Could you check a few things on this model? Use its own coordinates, in mm. A direction names the side the tool comes from. Give positions to 0.01 mm unless a question says otherwise; leave off trailing zeros. Order: outer loops, then holes, each group sorted by start corner. A loop starts at its lowest first (then second) coordinate and runs counter-clockwise, first axis right, second up. Notation, with made-up numbers: (86.5, -15.75) - (122.5, -15.75) arc R17 ccw to (122.5, -5.75) - close; hole circle Ø4 at (44, 57.25). An arc over 180 degrees is marked (long way). One line per question, with ' | ' between items. Start each with the question number.
1. Which directions (+Z, -Z, +X, -X, +Y, -Y) give clear straight access to the entire face, cutting with the end or side of a thin tool? Please do faces 4 (the cylindrical face through (-1.08, -4.88, 0.25)), 5 (the flat face through (6, 0, 3.5)), 6 (the cylindrical face through (-0.16, -9.76, 2.02)).
2. Imagine slicing it at A-A (z = 2). Give the number of separate pieces and of enclosed holes in the cut face, and give its area (3 significant figures).
3. For P1, Ø2, axis at x = -7.78, y = -7.78, coming from the +Z side (3 decimals); P2, Ø4, axis at x = 0, y = 11, coming from the -Z side; P3, Ø1, axis at x = -7, z = 1.5, coming from the +Y side; P4, Ø4, axis at x = -7.78, y = 7.78, coming from the +Z side, each with a flat end and sliding along its axis, tell me the tip position at first contact or that it passes through.
4. I need wall thicknesses on probe 1 along Y at (x, z) = (0, 2.4); probe 2 along X at (y, z) = (-8, 1.5); probe 3 along Y at (x, z) = (8.25, 3.25). Which ranges of each line are inside material? Lowest first, please. Write a range as from..to.
5. Imagine slicing it at D-D (z = 4.5). Please give me the cut outline in (x, y), and give its area (3 significant figures).
6. If we mould it in two halves opening along Y, with no side actions, what happens to faces 1 (the flat face through (0, 0, 8.5)), 2 (the cylindrical face through (-1.08, -4.88, 4.51)), 3 (the cylindrical face through (-9.76, 0.16, 2.02))? For each: released by +Y, released by -Y, zero draft, split by the parting line, or undercut.
```python
from build123d import *

# Parameters (mm, degrees)
SKETCH017_R           = 1.25
POCKET_DEPTH          = 3
POLARPATTERN_COUNT    = 8
SKETCH018_R           = 1
POCKET001_DEPTH       = 3
POLARPATTERN001_COUNT = 4
CHAMFER_SIZE          = 0.5
FILLET005_R           = 0.5


with BuildPart() as part:
    # Sketch016 → Revolution003 (revolve)
    with BuildSketch(Plane.XZ):
        Polygon((0, 0), (5, 0), (5, 0.5), (14, 0.5), (14, 3.5), (5, 3.5), (5, 5.5), (2.75, 5.5), (2.75, 8.5), (0, 8.5), align=None)
    revolve(axis=Axis((0, 0, 0), (0, 0, 1)))

    # Sketch017 (on Face5 of Revolution003) → Pocket (cut)
    with BuildSketch(Plane(origin=(0, 0, 3.5), x_dir=(-1, 0, 0), z_dir=(0, 0, 1))):
        with Locations((0, -11)):
            Circle(SKETCH017_R)
    pocket = extrude(amount=-POCKET_DEPTH, mode=Mode.SUBTRACT)

    # PolarPattern: Pocket ×8 about axis
    polarpattern_axis = Axis((0, 0, 3.5), (0, 0, 1))
    for i in range(1, POLARPATTERN_COUNT):
        add(pocket.rotate(polarpattern_axis, i * 360 / POLARPATTERN_COUNT), mode=Mode.SUBTRACT)

    # Sketch018 (on Face13 of PolarPattern) → Pocket001 (cut)
    with BuildSketch(Plane(origin=(0, 0, 3.5), x_dir=(-1, 0, 0), z_dir=(0, 0, 1))):
        with Locations((0, 8)):
            Circle(SKETCH018_R)
    pocket001 = extrude(amount=-POCKET001_DEPTH, mode=Mode.SUBTRACT)

    # PolarPattern001: Pocket001 ×4 about axis
    polarpattern001_axis = Axis((0, 0, 3.5), (0, 0, 1))
    for i in range(1, POLARPATTERN001_COUNT):
        add(pocket001.rotate(polarpattern001_axis, i * 360 / POLARPATTERN001_COUNT), mode=Mode.SUBTRACT)

    # Chamfer
    chamfer_edges = [part.edges().sort_by_distance(p)[0] for p in [
        (-14, 0, 3.5),
        (-14, 0, 0.5),
    ]]
    chamfer(chamfer_edges, length=CHAMFER_SIZE)

    # Fillet005
    fillet005_edges = [part.edges().sort_by_distance(p)[0] for p in [
        (-2.75, 0, 8.5),
    ]]
    fillet(fillet005_edges, radius=FILLET005_R)


solid = part.part
```
Results found:
1) face 4: -Z | face 5: +Z | face 6: +Z, -Z
2) separate pieces: 1 | enclosed holes: 12 | area: 564 mm2
3) P1: passes through | P2: stops at z = 0.5 | P3: stops at y = 12.4 | P4: stops at z = 3.5
4) probe 1: y = -14..-12.25, -9.75..-9, -7..7, 9..9.75, 12.25..14 | probe 2: x = -11.49..-9.01, -6.55..-1, 1..6.55, 9.01..11.49 | probe 3: y = -11..-8.94, -6.62..-0.97, 0.97..6.62, 8.94..11
5) outline: circle Ø10 at (0, 0) | area: 78.5 mm2
6) face 1: zero draft | face 2: split by the parting line | face 3: undercut
